Geometry: final body of the model. Coordinates: model frame, mm. A direction names the side the tool comes from. Coordinates: 2 decimals unless noted, no trailing zeros. Order: outer loops, then holes, each group sorted by start corner. A loop starts at its lowest first (then second) coordinate and runs counter-clockwise, first axis right, second up. Notation, with made-up numbers: (78, -30) - (98, -30) arc R29 cw to (98, 4) - close; hole circle Ø9 at (84.5, 13.5). An arc over 180 degrees is marked (long way). Use one line per item in the form item = value. Start each with the question number.
```python
from build123d import *


with BuildPart() as f2:
    # F2: sweep along a path in F1
    with BuildLine(Plane.YZ) as f2_path:
        Line((0, 0), (-254, 0))
        Line((-254, 0), (-343.8025612107, 89.8025612107))
        Line((-343.8025612107, 89.8025612107), (-343.8025612107, 166.0025612107))
    # F0 (on Front) → F2 (sweep)
    with BuildSketch(Plane.XZ):
        Polygon((-88.9, 12.7), (-88.9, 0), (0, 0), (0, 12.7), (-38.1, 12.7), (-38.1, 45.72), (0, 45.72), (0, 58.42), (-88.9, 58.42), (-88.9, 45.72), (-50.8, 45.72), (-50.8, 12.7), align=None)
    sweep(path=f2_path.line, transition=Transition.RIGHT)

    # F2_face (on face) → F5 section 0
    with BuildSketch(Plane(origin=(-44.45, 0, 29.21), x_dir=(-1, 0, 0), z_dir=(0, 1, 0))):
        Polygon((44.45, -16.51), (6.35, -16.51), (6.35, 16.51), (44.45, 16.51), (44.45, 29.21), (-44.45, 29.21), (-44.45, 16.51), (-6.35, 16.51), (-6.35, -16.51), (-44.45, -16.51), (-44.45, -29.21), (44.45, -29.21), align=None)
    # F4 (on offset) → F5 section 1
    with BuildSketch(Plane.XZ.offset(-254)):
        Polygon((-88.9, 0), (0, 0), (0, 6.35), (-6.35, 6.35), (-6.35, 52.07), (0, 52.07), (0, 58.42), (-88.9, 58.42), (-88.9, 52.07), (-82.55, 52.07), (-82.55, 6.35), (-88.9, 6.35), align=None)
    loft()


solid = f2.part
```
(1) Cut plane B-B on y = -90. Return the cut outline in (x, z), plus the area to 3 significant figures.
(2) Cut plane A-A on z = 148.5. Return the cut outline in (x, y).
(3) Set-up query: faces 1 (the flat face through (-45, 15, 58.42)), 2 (the flat face through (-19, -331.103, 131)), 3 (the flat face through (-70, -331.103, 131)). Return all of +Z, -Z, +X, -X, +Y, -Y with unobstructed straight access to the full face (end or side cutting, diameter ignored); none if empty.
(4) Material intervals for L1, parallel to Z at x = -36, y = -143; L2, parallel to Y at x = -83.5, z = 149; L3, parallel to Z at x = -44.5, y = 216, sorted ascending. Write a range as from..to.
(5) Contact query for flat-ended pins moving along their axis: pin 1 Ø8 at (x, z) = (-28, 105) entering from +Y; pin 2 Ø12 at (x, y) = (-78.5, 166.5) entering from +Z; pin 3 Ø12 at (x, z) = (-20, 108) entering from +Y; pin 4 Ø10 at (x, y) = (-51.5, 59) entering from -Z. Output: stop coordinate, or through.
Check sheet entries:
q1.outline = (-88.9, 0) - (0, 0) - (0, 12.7) - (-38.1, 12.7) - (-38.1, 45.72) - (0, 45.72) - (0, 58.42) - (-88.9, 58.42) - (-88.9, 45.72) - (-50.8, 45.72) - (-50.8, 12.7) - (-88.9, 12.7) - close
q1.area = 2,680 mm^2
q2.outline = (-88.9, -343.8) - (0, -343.8) - (0, -331.1) - (-38.1, -331.1) - (-38.1, -298.08) - (0, -298.08) - (0, -285.38) - (-88.9, -285.38) - (-88.9, -298.08) - (-50.8, -298.08) - (-50.8, -331.1) - (-88.9, -331.1) - close
q3.face_1 = +Z, +X, -X, +Y
q3.face_2 = +Z, +X
q3.face_3 = +Z, -X
q4.L1 = 0..12.7, 45.72..58.42
q4.L2 = -343.8..-331.1, -298.08..-285.38
q4.L3 = 0..58.42
q5.pin_1 = -272.38
q5.pin_2 = 58.42
q5.pin_3 = -273.38
q5.pin_4 = 0
